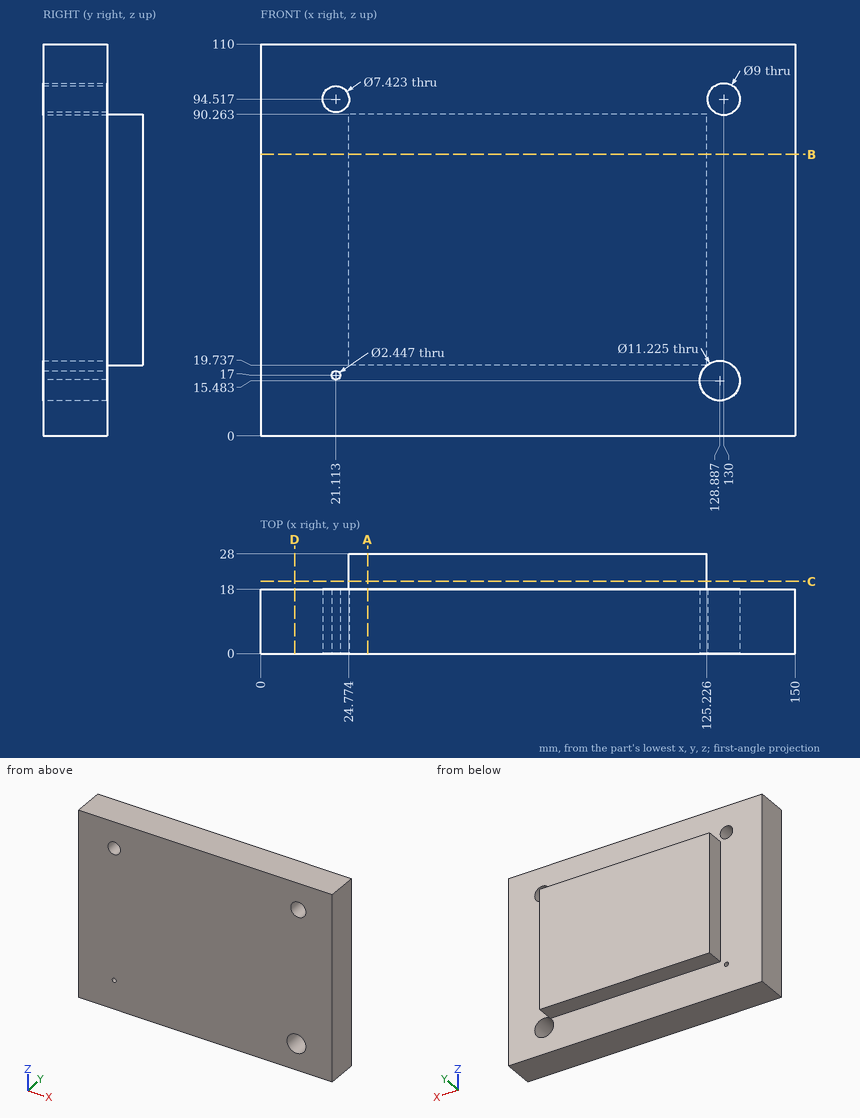
The drawing under review shows one solid part. Ordinate dimensions are in mm from its lowest x, y, z. Coordinates: 2 decimals unless noted, no trailing zeros. Order: outer loops, then holes, each group sorted by start corner. A loop starts at its lowest first (then second) coordinate and runs counter-clockwise, first axis right, second up. Notation, with made-up numbers: (66.25, 15) -> (81.25, 15) arc R15 cw to (81.25, 43) -> close; hole circle Ø2 at (-3, -2). An arc over 180 degrees is marked (long way). Answer as CSV lines item,"result".
Q1. Clearance check with flat-ended pins moving along their axes: pin 1 Ø1.5 at (y, z) = (22, 49.5) entering from +X; pin 2 Ø5 at (x, y) = (25.5, 19) entering from -Z; pin 3 Ø5 at (x, y) = (81, 23) entering from +Z; pin 4 Ø2 at (x, y) = (38, 19.5) entering from -Z. State where each tip first meets the part, or that it passes through.
Model answer:
pin 1,"stops at x = 125.23"
pin 2,"stops at z = 0"
pin 3,"stops at z = 90.26"
pin 4,"stops at z = 19.74"
Q2. We need section A-A (x = 30). State the section outline as (y, z) points.
Model answer:
outline,"(0, 0) -> (18, 0) -> (18, 19.74) -> (28, 19.74) -> (28, 90.26) -> (18, 90.26) -> (18, 110) -> (0, 110) -> close"
Q3. We need section C-C (y = 20.25). State the section outline as (x, z) points, plus the area to 3 significant figures.
Model answer:
outline,"(24.77, 19.74) -> (125.23, 19.74) -> (125.23, 90.26) -> (24.77, 90.26) -> close"
area,"7,080 mm2"
Q4. We need section D-D (x = 9.5). State the section outline as (y, z) points.
Model answer:
outline,"(0, 0) -> (18, 0) -> (18, 110) -> (0, 110) -> close"
Q5. Wall thickness on line 1 along Z through (x, y) = (129.5, 12) (1 decimal); line 2 along Z through (x, y) = (87.5, 22.5); line 3 along Y through (x, z) = (67, 99): over which ranges is each line inside the solid? List them lowest first. Write a range as [from, to].
Model answer:
line 1,"z = [0, 9.9], [21.1, 90], [99, 110]"
line 2,"z = [19.74, 90.26]"
line 3,"y = [0, 18]"
Q6. We need section B-B (z = 79). State the section outline as (x, y) points.
Model answer:
outline,"(0, 0) -> (150, 0) -> (150, 18) -> (125.23, 18) -> (125.23, 28) -> (24.77, 28) -> (24.77, 18) -> (0, 18) -> close"
